from build123d import *

# Parameters (mm, degrees)
F0_W     = 90
F0_H     = 140
F0_W_2   = 60
F0_H_2   = 15
F1_DEPTH = 5
F2_W     = 82
F2_H     = 132
F2_W_2   = 70
F2_H_2   = 120
F3_DEPTH = 12
F4_R     = 2.25
F5_DEPTH = 86.001
F6_R     = 2.25
F7_DEPTH = 136.001
F8_W     = 70
F8_H     = 12
F8_R     = 2.25
F9_DEPTH = 6


with BuildPart() as f1:
    # F0 (on Top) → F1 (new body)
    with BuildSketch(Plane.XY):
        Rectangle(F0_W, F0_H)
        Polygon((-30, 32.5), (-30, 55), (-7.5, 55), (7.5, 55), (30, 55), (30, 32.5), (30, 17.5), (30, 7.5), (30, -7.5), (30, -17.5), (30, -32.5), (30, -55), (7.5, -55), (-7.5, -55), (-30, -55), (-30, -32.5), (-30, -17.5), (-30, -7.5), (-30, 7.5), (-30, 17.5), align=None, mode=Mode.SUBTRACT)
        Polygon((7.5, 55), (-7.5, 55), (-30, 32.5), (-30, 17.5), (0, 47.5), (30, 17.5), (30, 32.5), align=None)
        Polygon((0, -47.5), (-30, -17.5), (-30, -32.5), (-7.5, -55), (7.5, -55), (30, -32.5), (30, -17.5), align=None)
        Rectangle(F0_W_2, F0_H_2)
    extrude(amount=F1_DEPTH)

    # F2 (on face) → F3 (join)
    with BuildSketch(Plane.XY.offset(5)):
        Rectangle(F2_W, F2_H)
        Rectangle(F2_W_2, F2_H_2, mode=Mode.SUBTRACT)
    extrude(amount=F3_DEPTH)

    # F4 (on face) → F5 (cut, through all)
    with BuildSketch(Plane(origin=(-41, 0, 0), x_dir=(0, -1, 0), z_dir=(-1, 0, 0))):
        with Locations((-50, 11)):
            Circle(F4_R)
        with Locations((0, 11)):
            Circle(F4_R)
        with Locations((50, 11)):
            Circle(F4_R)
    extrude(amount=-F5_DEPTH, mode=Mode.SUBTRACT)

    # F6 (on face) → F7 (cut, through all)
    with BuildSketch(Plane(origin=(0, 66, 0), x_dir=(-1, 0, 0), z_dir=(0, 1, 0))):
        with Locations((-30, 11)):
            Circle(F6_R)
        with Locations((0, 11)):
            Circle(F6_R)
        with Locations((30, 11)):
            Circle(F6_R)
    extrude(amount=-F7_DEPTH, mode=Mode.SUBTRACT)

    # F8 (on face) → F9 (cut, through all)
    with BuildSketch(Plane(origin=(0, 66, 0), x_dir=(-1, 0, 0), z_dir=(0, 1, 0))):
        with Locations((0, 11)):
            Rectangle(F8_W, F8_H)
        with Locations((-30, 11)):
            Circle(F8_R, mode=Mode.SUBTRACT)
        with Locations((0, 11)):
            Circle(F8_R, mode=Mode.SUBTRACT)
        with Locations((30, 11)):
            Circle(F8_R, mode=Mode.SUBTRACT)
    extrude(amount=-F9_DEPTH, mode=Mode.SUBTRACT)


solid = f1.part
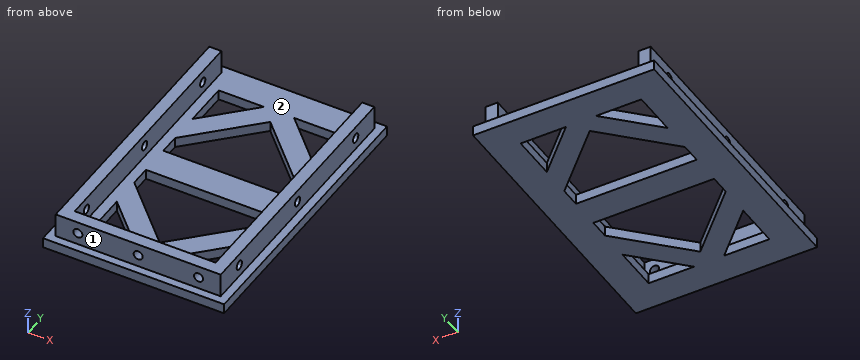
Geometry check sheet. Reference: the model listing, model coordinates, mm. Face numbers are marked on the shaded views. Give positions to 0.01 mm unless a question says otherwise; leave off trailing zeros. Write each loop counter-clockwise with the first axis right and the second up, starting at its lowest first coordinate (ties: lowest second). Pieces come first, ordered by that corner, then holes. Notation, with made-up numbers: (67.25, 75.5) - (82.25, 75.5) arc R18 cw to (82.25, 99.5) - close; hole circle Ø7 at (37.5, 24.5). An arc over 180 degrees is marked (long way). Put each result on its own line as item: value.
1. Sectioned sample at C-C, the plane y = 0. Enter the section's corners in (x, z).
Ans:
outline: (-45, 0) - (45, 0) - (45, 5) - (41, 5) - (41, 8.75) - (35, 8.75) - (35, 5) - (-35, 5) - (-35, 8.75) - (-41, 8.75) - (-41, 5) - (-45, 5) - close; (-41, 13.25) - (-35, 13.25) - (-35, 17) - (-41, 17) - close; (35, 13.25) - (41, 13.25) - (41, 17) - (35, 17) - close
2. Sectioned sample at B-B, the plane y = -26. Enter the section's corners in (x, z), plus the area to 3 significant figures.
Ans:
outline: (-45, 0) - (-21.5, 0) - (-21.5, 5) - (-35, 5) - (-35, 17) - (-41, 17) - (-41, 5) - (-45, 5) - close; (21.5, 0) - (45, 0) - (45, 5) - (41, 5) - (41, 17) - (35, 17) - (35, 5) - (21.5, 5) - close
area: 379 mm²
3. Sectioned sample at A-A, the plane x = 18. Enter the section's corners in (y, z), plus the area to 3 significant figures.
Ans:
outline: (-70, 0) - (-55, 0) - (-55, 5) - (-60, 5) - (-60, 17) - (-66, 17) - (-66, 5) - (-70, 5) - close; (-44.5, 0) - (-29.5, 0) - (-29.5, 5) - (-44.5, 5) - close; (-7.5, 0) - (7.5, 0) - (7.5, 5) - (-7.5, 5) - close; (29.5, 0) - (44.5, 0) - (44.5, 5) - (29.5, 5) - close; (55, 0) - (70, 0) - (70, 5) - (55, 5) - close
area: 447 mm²
4. Sectioned sample at D-D, the plane z = 2.5. Enter the section's corners in (x, y), plus the area to 3 significant figures.
Ans:
outline: (-45, -70) - (45, -70) - (45, 70) - (-45, 70) - close; hole (-30, -55) - (-7.5, -55) - (-30, -32.5) - close; hole (-30, -17.5) - (0, -47.5) - (30, -17.5) - (30, -7.5) - (-30, -7.5) - close; hole (-30, 7.5) - (30, 7.5) - (30, 17.5) - (0, 47.5) - (-30, 17.5) - close; hole (-30, 32.5) - (-7.5, 55) - (-30, 55) - close; hole (7.5, -55) - (30, -55) - (30, -32.5) - close; hole (7.5, 55) - (30, 32.5) - (30, 55) - close
area: 8,590 mm²
5. Thickness scan on line 1 (Y direction, x = 0, z = 4); line 2 (X direction, y = 38, z = 7.5); line 3 (Z direction, x = -37, y = 50). Record the ranges inside material, lowest first.
Ans:
line 1: y = -70 to -47.5, -7.5 to 7.5, 47.5 to 70
line 2: x = -41 to -35, 35 to 41
line 3: z = 0 to 8.75, 13.25 to 17
6. Go/stop test with flat-tipped pins: pin 1 (2 mm diameter, centred on x = 7, z = 9.5, fed in from +Y); pin 2 (5 mm diameter, centred on y = 0, z = 11, fed in from +X); pin 3 (3.5 mm diameter, centred on y = 0, z = 11, fed in from +X); pin 4 (3 mm diameter, centred on x = 1, z = 11, fed in from -Y). Record where each tip stops, or that it passes through.
Ans:
pin 1: stops at y = -60
pin 2: stops at x = 41
pin 3: passes through
pin 4: stops at y = -66
7. Draft check along X on the marked faces 1 and 2. Enter one of: +X half, -X half, draft (parallel to the pull), parting line (faces both ways), or undercut.
Ans:
face 1: draft
face 2: undercut
